```python
from build123d import *

# Parameters (mm, degrees)
SKETCH1_R           = 24
BOSS_EXTRUDE1_DEPTH = 1
SKETCH3_R           = 2.1
CUT_EXTRUDE2_DEPTH  = 2
SKETCH2_R           = 1.6
CUT_EXTRUDE3_DEPTH  = 2
SKETCH4_W           = 0.94378815
SKETCH4_H           = 0.65487341
CUT_EXTRUDE4_DEPTH  = 0.3


with BuildPart() as part:
    # Sketch1 → Boss-Extrude1 (new body)
    with BuildSketch(Plane.XY):
        Circle(SKETCH1_R)
    extrude(amount=BOSS_EXTRUDE1_DEPTH)

    # Sketch3 → Cut-Extrude2 (cut)
    with BuildSketch(Plane.XY.offset(1)):
        Circle(SKETCH3_R)
    extrude(amount=-CUT_EXTRUDE2_DEPTH, mode=Mode.SUBTRACT)

    # Sketch2 → Cut-Extrude3 (cut, through all)
    with BuildSketch(Plane.XY.offset(1)):
        with Locations((-18, 0)):
            Circle(SKETCH2_R)
        with Locations((0, 18)):
            Circle(SKETCH2_R)
        with Locations((18, 0)):
            Circle(SKETCH2_R)
        with Locations((0, -18)):
            Circle(SKETCH2_R)
    extrude(amount=-CUT_EXTRUDE3_DEPTH, mode=Mode.SUBTRACT)

    # Sketch4 → Cut-Extrude4 (cut)
    with BuildSketch(Plane.XY.offset(1)):
        Polygon((-11.58574855, 12.841946562), (-8.291473373, 12.841946562), (-10.597161191, 9.019905494), (-11.751924249, 9.019905494), (-9.607705981, 12.052611994), (-11.58574855, 12.052611994), align=None)
        Polygon((-13.559084971, 12.841946562), (-16.044695483, 12.841946562), (-16.044695483, 10.889382104), (-14.639227012, 10.889382104), (-14.639227012, 9.019905494), (-13.559084971, 9.019905494), align=None)
        with Locations((-14.783101119, 12.008686539)):
            Rectangle(SKETCH4_W, SKETCH4_H, mode=Mode.SUBTRACT)
    extrude(amount=-CUT_EXTRUDE4_DEPTH, mode=Mode.SUBTRACT)


solid = part.part
```
Here's how the part is built. I have some questions about the finished solid (model axes, mm). Coordinates: 2 decimals unless noted, no trailing zeros. Write each loop counter-clockwise with the first axis right and the second up, starting at its lowest first coordinate (ties: lowest second). Pieces come first, ordered by that corner, then holes. Notation, with made-up numbers: (15.5, 46) -> (52.5, 46) arc R16 cw to (52.5, 69) -> close; hole circle Ø11 at (22.25, 67.5). An arc over 180 degrees is marked (long way). Use a Markdown table: item, result. Add a question column.
(1) I'm going to push flat-ended pins straight in: P1, Ø3.5, axis at x = -18, y = 0, coming from the -Z side; P2, Ø2.5, axis at x = 0, y = 18, coming from the -Z side (1 decimal). Where does each tip first touch, or does it pass through?
(2) We'd pull the mould along Y, two halves only. Please class faces 1 (the cylindrical face through (-23.977, 1.055, 0.493)), 2 (the cylindrical face through (-0.208, 19.586, 0.507)), 3 (the cylindrical face through (-19.6, 0.07, 0.51)), 4 (the flat face through (5, 0, 1)): +Y half, -Y half, draft (parallel to the pull), parting line (faces both ways), or undercut.
(3) Please list where these lines run through material, in increasing order: line 1 (Y direction, x = 0, z = 0.35); line 2 (X direction, y = 10, z = 0.9); line 3 (Y direction, x = -17, z = 0.3).
(4) If we section it at C-C, the plane y = -18: Write out the boundary of the cut face in (x, z), and give its area (3 significant figures).
(5) If we section it at A-A, the plane x = 0: Write out the boundary of the cut face in (y, z), and give its area (3 significant figures).
Outcome:
| question | item | result |
|---|---|---|
| 1 | P1 | stops at z = 0 |
| 1 | P2 | passes through |
| 2 | face 1 | parting line |
| 2 | face 2 | undercut |
| 2 | face 3 | undercut |
| 2 | face 4 | draft |
| 3 | line 1 | y = -24 to -19.6, -16.4 to -2.1, 2.1 to 16.4, 19.6 to 24 |
| 3 | line 2 | x = -21.82 to -14.64, -13.56 to -11.06, -10.01 to 21.82 |
| 3 | line 3 | y = -16.94 to -1.25, 1.25 to 16.94 |
| 4 | outline | (-15.87, 0) -> (-1.6, 0) -> (-1.6, 1) -> (-15.87, 1) -> close; (1.6, 0) -> (15.87, 0) -> (15.87, 1) -> (1.6, 1) -> close |
| 4 | area | 28.5 mm^2 |
| 5 | outline | (-24, 0) -> (-19.6, 0) -> (-19.6, 1) -> (-24, 1) -> close; (-16.4, 0) -> (-2.1, 0) -> (-2.1, 1) -> (-16.4, 1) -> close; (2.1, 0) -> (16.4, 0) -> (16.4, 1) -> (2.1, 1) -> close; (19.6, 0) -> (24, 0) -> (24, 1) -> (19.6, 1) -> close |
| 5 | area | 37.4 mm^2 |
